Could you check a few things on this model? Use its own coordinates, in mm. A direction names the side the tool comes from. Give positions to 0.01 mm unless a question says otherwise; leave off trailing zeros. Order: outer loops, then holes, each group sorted by start corner. A loop starts at its lowest first (then second) coordinate and runs counter-clockwise, first axis right, second up. Notation, with made-up numbers: M 77.25,36 L 129.25,36 A12 ccw 129.25,54 Z; hole C -38.75,63.5 d4. An arc over 180 degrees is marked long. Use a Markdown table: item, result. Add a question column.
Item 1: If I drill on L1, parallel to X at y = -21.5, z = 0; L2, parallel to Z at x = 0, y = -12; L3, parallel to X at y = 6.5, z = 20.5, over which ranges is the centre line in solid material (lowest first)? Write a range as from..to.
Item 2: If we mould it in two halves opening along Z, with no side actions, what happens to faces 4 (the face through (-55, -50, -1)), 5 (the face through (47.69, -0.7, -15.02)), 6 (the face through (158.038, 9.175, -11.966)), 7 (the face through (157.446, -3.522, 11.183))? For each: released by +Z, released by -Z, zero draft, split by the parting line, or undercut.
Item 3: Suppose I cut it at D-D on x = 82.5. Write out the boundary of the cut face in (y, z), plus the area to 3 significant figures.
Item 4: I'm going to push flat-ended pins straight in: pin 1 Ø3 at (y, z) = (-4, 15) entering from +X; pin 2 Ø12 at (x, y) = (29, -10) entering from -Z; pin 3 Ø3 at (x, z) = (114.5, 26.5) entering from -Y. Where does each tip first touch, or does it pass through?
Item 5: Suppose I cut it at A-A on x = 0. Write out the boundary of the cut face in (y, z), plus the area to 3 significant figures.
Item 6: Suppose I cut it at C-C on y = -36. Write out the boundary of the cut face in (x, z).
Item 7: For faces 1 (the face through (-80, 1, 1)), 2 (the face through (134, 11, 17)), 3 (the face through (149, 17, 7)), which set-ups out of +Z, -Z, +X, -X, +Y, -Y let a thin tool reach every point of the face, with its end or its side?
Item 8: Suppose I cut it at B-B on z = 29. Write out the boundary of the cut face in (x, y).
from build123d import *

# Parameters (mm, degrees)
SKETCH1_R           = 50
BOSS_EXTRUDE1_DEPTH = 50
BOSS_EXTRUDE2_REACH = 202
SKETCH2_R           = 45


with BuildPart() as part:
    # Sketch1 → Boss-Extrude1 (new body, symmetric)
    with BuildSketch(Plane(origin=(0, 0, 0), x_dir=(1, 0, 0), z_dir=(0, 1, 0))):
        with BuildLine():
            Line((-80, -40), (-80, 40))
            Line((-80, 40), (-16.407423315, 62.895122706))
            ThreePointArc((-16.407423315, 62.895122706), (65, 0), (-16.407423315, -62.895122706))
            Line((-16.407423315, -62.895122706), (-80, -40))
        make_face()
        Circle(SKETCH1_R, mode=Mode.SUBTRACT)
    extrude(amount=BOSS_EXTRUDE1_DEPTH, both=True)

    # Sketch2 → Boss-Extrude2 (add, up to next)
    with BuildSketch(Plane(origin=(120, 0, 0), x_dir=(0, 0, -1), z_dir=(1, 0, 0)), mode=Mode.PRIVATE) as boss_extrude2_sk1:
        Circle(SKETCH2_R)
    boss_extrude2_tool1 = extrude(boss_extrude2_sk1.sketch, amount=-BOSS_EXTRUDE2_REACH, mode=Mode.PRIVATE) - part.part
    add(boss_extrude2_tool1.solids().sort_by_distance((120, 0, 0))[0])

    # Sketch3 → Revolve1 (revolve)
    with BuildSketch(Plane(origin=(0, 0, 0), x_dir=(1, 0, 0), z_dir=(0, 1, 0))):
        Polygon((120, 0), (120, -20), (134, -20), (134, -25.051306185), (149, -25.051306185), (149, -18.051306185), (158.499342873, -14.926808627), (157.392152325, -11.560640965), (192.539720953, 0), align=None)
    revolve(axis=Axis((0, 0, 0), (1, 0, 0)))


solid = part.part
Findings below:
| question | item | result |
|---|---|---|
| 1 | L1 | x = -80..-50, 50..120, 134..149 |
| 1 | L2 | z = -65..-50, 50..65 |
| 1 | L3 | x = -80..-45.6, 45.6..120, 134..149 |
| 2 | face 4 | zero draft |
| 2 | face 5 | undercut |
| 2 | face 6 | split by the parting line |
| 2 | face 7 | undercut |
| 3 | outline | C 0,0 d90 |
| 3 | area | 6,360 mm^2 |
| 4 | pin 1 | stops at x = 158.5 |
| 4 | pin 2 | stops at z = -60.79 |
| 4 | pin 3 | stops at y = -37.42 |
| 5 | outline | M -50,-65 L 50,-65 L 50,-50 L -50,-50 Z; M -50,50 L 50,50 L 50,65 L -50,65 Z |
| 5 | area | 3,000 mm^2 |
| 6 | outline | M -80,-40 L -16.41,-62.9 A65 ccw 59.13,-27 L 120,-27 L 120,27 L 59.13,27 A65 ccw -16.41,62.9 L -80,40 Z; hole C 0,0 d100 |
| 7 | face 1 | +Z, -Z, -X, +Y, -Y |
| 7 | face 2 | none |
| 7 | face 3 | +X |
| 8 | outline | M -80,-50 L -40.73,-50 L -40.73,50 L -80,50 Z; M 40.73,-50 L 58.17,-50 L 58.17,-34.41 L 120,-34.41 L 120,34.41 L 58.17,34.41 L 58.17,50 L 40.73,50 Z |
